Source: three-view drawing plus pictorial views. Frame: mm from the lowest corner of the part. A direction names the side the tool comes from. Give positions to 0.01 mm unless a question says otherwise; leave off trailing zeros. Loops run counter-clockwise (first coordinate to the right, second up) from the corner with the lowest first, then second, coordinate; pieces in that order, holes last. Notation, with made-up numbers: (-30, -35) - (24, -35) arc R25 ccw to (24, -5) - close; hole circle Ø6 at (56.25, -25). An arc over 180 degrees is marked (long way). Answer in a Markdown table with one row per item.
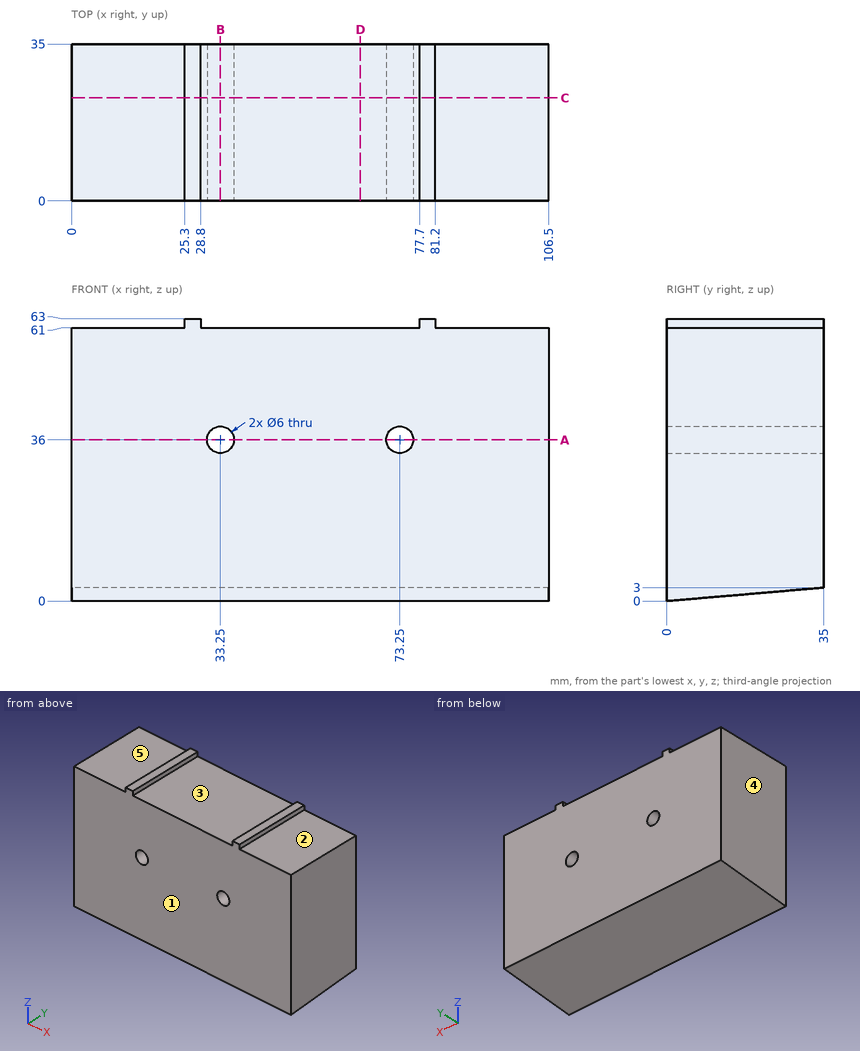
Q1. First-contact query: pin 1 (10 mm diameter, centred on x = 48, z = 20.5, fed in from -Y); pin 2 (1 mm diameter, centred on y = 26, z = 62, fed in from +X); pin 3 (5.5 mm diameter, centred on x = 73.25, z = 36, fed in from -Y); pin 4 (0.6 mm diameter, centred on y = 14, z = 61.5, fed in from -X). Flat tips, straight axial feed; report the tip coordinate or a pass-through.
Check values:
| item | result |
|---|---|
| pin 1 | y = 0 |
| pin 2 | x = 81.2 |
| pin 3 | through |
| pin 4 | x = 25.3 |
Q2. Cut plane C-C (y = 23). Output: boundary loops of the cut face in (x, z).
Check values:
| item | result |
|---|---|
| outline | (0, 1.97) - (106.5, 1.97) - (106.5, 61) - (81.2, 61) - (81.2, 63) - (77.7, 63) - (77.7, 61) - (28.8, 61) - (28.8, 63) - (25.3, 63) - (25.3, 61) - (0, 61) - close; hole circle Ø6 at (33.25, 36); hole circle Ø6 at (73.25, 36) |
Q3. Material intervals for line 1 along X through (y, z) = (18, 36); line 2 along Z through (x, y) = (73.25, 19.5); line 3 along Z through (x, y) = (33, 9), sorted ascending.
Check values:
| item | result |
|---|---|
| line 1 | 0 to 30.25, 36.25 to 70.25, 76.25 to 106.5 |
| line 2 | 1.67 to 33, 39 to 61 |
| line 3 | 0.77 to 33.01, 38.99 to 61 |
Q4. Cut plane D-D (x = 64.5). Output: boundary loops of the cut face in (y, z), and give its area (3 significant figures).
Check values:
| item | result |
|---|---|
| outline | (0, 0) - (35, 3) - (35, 61) - (0, 61) - close |
| area | 2,080 mm² |
Q5. Cut plane B-B (x = 33.25). Output: boundary loops of the cut face in (y, z), and give its area (3 significant figures).
Check values:
| item | result |
|---|---|
| outline | (0, 0) - (35, 3) - (35, 33) - (0, 33) - close; (0, 39) - (35, 39) - (35, 61) - (0, 61) - close |
| area | 1,870 mm² |
Q6. Reachability of the marked faces 1 and 2 from +Z, -Z, +X, -X, +Y, -Y: full face, straight path, thin tool, end or side. Return the list, or none.
Check values:
| item | result |
|---|---|
| face 1 | +Z, -Z, +X, -X, -Y |
| face 2 | +Z, +X, +Y, -Y |
Q7. Draft query along X for the marked faces 3, 4 and 5. Return one class per face: pulls with the +X half, pulls with the -X half, needs draft (parallel to the pull), parting line crosses it, or undercut.
Check values:
| item | result |
|---|---|
| face 3 | undercut |
| face 4 | pulls with the -X half |
| face 5 | needs draft |
Q8. Cut plane A-A (z = 36). Output: boundary loops of the cut face in (x, y), and give its area (3 significant figures).
Check values:
| item | result |
|---|---|
| outline | (0, 0) - (30.25, 0) - (30.25, 35) - (0, 35) - close; (36.25, 0) - (70.25, 0) - (70.25, 35) - (36.25, 35) - close; (76.25, 0) - (106.5, 0) - (106.5, 35) - (76.25, 35) - close |
| area | 3,310 mm² |
